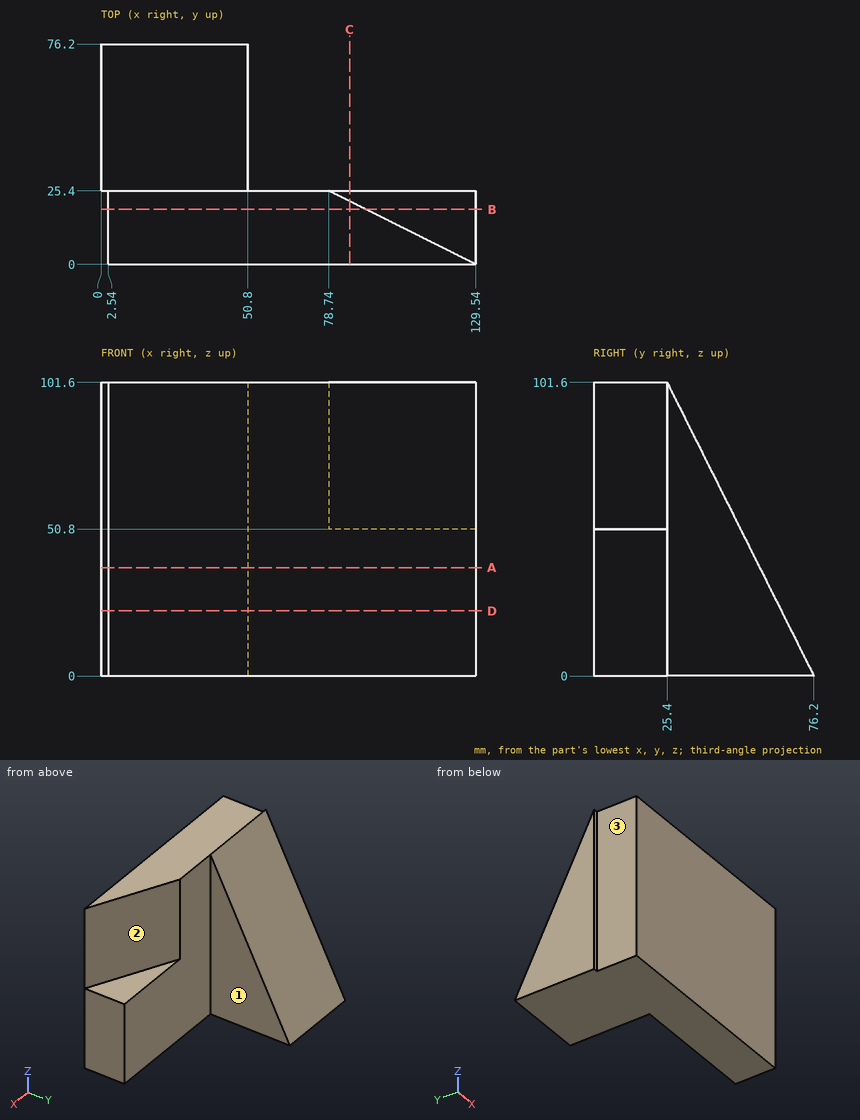
Can you work these out from the drawing? Everything is in mm from the part's minimum corner. A direction names the side the tool comes from. Give positions to 0.01 mm unless a question says otherwise; leave off trailing zeros. Loops run counter-clockwise (first coordinate to the right, second up) from the corner with the lowest first, then second, coordinate; pieces in that order, holes last. Notation, with made-up numbers: (-25, 29) - (31, 29) arc R14 cw to (31, 39) - close; hole circle Ø3 at (62.25, 3.5). An arc over 180 degrees is marked (long way). Answer as a JSON object with one key per item and string values.
Q1. Imagine slicing it at A-A on z = 37.5. Write out the boundary of the cut face in (x, y), plus the area to 3 significant figures.
Geometry says:
{"outline": "(0, 25.4) - (2.54, 25.4) - (2.54, 0) - (129.54, 0) - (129.54, 25.4) - (50.8, 25.4) - (50.8, 57.45) - (0, 57.45) - close", "area": "4,850 mm²"}
Q2. Imagine slicing it at C-C on x = 86. Write out the boundary of the cut face in (y, z), plus the area to 3 significant figures.
Geometry says:
{"outline": "(0, 0) - (25.4, 0) - (25.4, 50.8) - (21.77, 50.8) - (21.77, 101.6) - (0, 101.6) - close", "area": "2,400 mm²"}
Q3. Imagine slicing it at B-B on y = 19. Write out the boundary of the cut face in (x, z), plus the area to 3 significant figures.
Geometry says:
{"outline": "(2.54, 0) - (129.54, 0) - (129.54, 50.8) - (91.54, 50.8) - (91.54, 101.6) - (2.54, 101.6) - close", "area": "11,000 mm²"}
Q4. If I drill on L1, parallel to Y at x = 76, z = 91; L2, parallel to Z at x = 106, y = 24, over which ranges is the centre line in solid material (lowest first)?
Geometry says:
{"L1": "0 to 25.4", "L2": "0 to 50.8"}
Q5. Imagine slicing it at D-D on z = 22.5. Write out the boundary of the cut face in (x, y).
Geometry says:
{"outline": "(0, 25.4) - (2.54, 25.4) - (2.54, 0) - (129.54, 0) - (129.54, 25.4) - (50.8, 25.4) - (50.8, 64.95) - (0, 64.95) - close"}
Q6. Will these pins go through, and if not, where does the flat tip stop? P1, Ø4, axis at x = 37, y = 37.5, coming from the +Z side; P2, Ø2, axis at x = 1.5, z = 35.5, coming from the -Y side; P3, Ø5, axis at y = 42, z = 68, coming from the +X side.
Geometry says:
{"P1": "z = 81.4", "P2": "y = 25.4", "P3": "x = 50.8"}
Q7. Which directions (+Z, -Z, +X, -X, +Y, -Y) give clear straight access to the entire face, cutting with the end or side of a thin tool? Please do the marked faces 1, 2 and 3.
Geometry says:
{"face 1": "+Z, -Z, +X, +Y", "face 2": "+Z, +X, +Y", "face 3": "+Z, -Z, -X, -Y"}
